The model under review builds one solid part; all positions refer to its coordinate system, in mm. Coordinates: 2 decimals unless noted, no trailing zeros. Order: outer loops, then holes, each group sorted by start corner. A loop starts at its lowest first (then second) coordinate and runs counter-clockwise, first axis right, second up. Notation, with made-up numbers: M -5.75,87.25 L 20.25,87.25 A19 ccw 20.25,93.25 Z; hole C 40,84.5 d7. An arc over 180 degrees is marked long. One line per item, written item: value.
```python
from build123d import *

# Parameters (mm, degrees)
F0_R     = 8.5
F1_DEPTH = 3


with BuildPart() as f1:
    # F0 (on Front) → F1 (new body)
    with BuildSketch(Plane.XZ):
        with BuildLine():
            ThreePointArc((0, 55), (16.109127, 16.109127), (55, 0))
            Line((55, 0), (305, 0))
            ThreePointArc((305, 0), (315.606602, 4.393398), (320, 15))
            Line((320, 15), (320, 100))
            ThreePointArc((320, 100), (315.606602, 110.606602), (305, 115))
            Line((305, 115), (15, 115))
            ThreePointArc((15, 115), (4.393398, 110.606602), (0, 100))
            Line((0, 100), (0, 55))
        make_face()
        with Locations((75, 20)):
            Circle(F0_R, mode=Mode.SUBTRACT)
        with Locations((100, 20)):
            Circle(F0_R, mode=Mode.SUBTRACT)
        with Locations((125, 20)):
            Circle(F0_R, mode=Mode.SUBTRACT)
        with Locations((150, 20)):
            Circle(F0_R, mode=Mode.SUBTRACT)
        with Locations((75, 45)):
            Circle(F0_R, mode=Mode.SUBTRACT)
        with Locations((100, 45)):
            Circle(F0_R, mode=Mode.SUBTRACT)
        with Locations((125, 45)):
            Circle(F0_R, mode=Mode.SUBTRACT)
        with Locations((150, 45)):
            Circle(F0_R, mode=Mode.SUBTRACT)
        with Locations((175, 20)):
            Circle(F0_R, mode=Mode.SUBTRACT)
        with Locations((200, 20)):
            Circle(F0_R, mode=Mode.SUBTRACT)
        with Locations((225, 20)):
            Circle(F0_R, mode=Mode.SUBTRACT)
        with Locations((250, 20)):
            Circle(F0_R, mode=Mode.SUBTRACT)
        with Locations((275, 20)):
            Circle(F0_R, mode=Mode.SUBTRACT)
        with Locations((300, 20)):
            Circle(F0_R, mode=Mode.SUBTRACT)
        with Locations((175, 45)):
            Circle(F0_R, mode=Mode.SUBTRACT)
        with Locations((200, 45)):
            Circle(F0_R, mode=Mode.SUBTRACT)
        with Locations((225, 45)):
            Circle(F0_R, mode=Mode.SUBTRACT)
        with Locations((250, 45)):
            Circle(F0_R, mode=Mode.SUBTRACT)
        with Locations((275, 45)):
            Circle(F0_R, mode=Mode.SUBTRACT)
        with Locations((300, 45)):
            Circle(F0_R, mode=Mode.SUBTRACT)
        with Locations((75, 70)):
            Circle(F0_R, mode=Mode.SUBTRACT)
        with Locations((100, 70)):
            Circle(F0_R, mode=Mode.SUBTRACT)
        with Locations((125, 70)):
            Circle(F0_R, mode=Mode.SUBTRACT)
        with Locations((150, 70)):
            Circle(F0_R, mode=Mode.SUBTRACT)
        with Locations((100, 95)):
            Circle(F0_R, mode=Mode.SUBTRACT)
        with Locations((125, 95)):
            Circle(F0_R, mode=Mode.SUBTRACT)
        with Locations((150, 95)):
            Circle(F0_R, mode=Mode.SUBTRACT)
        with Locations((175, 70)):
            Circle(F0_R, mode=Mode.SUBTRACT)
        with Locations((200, 70)):
            Circle(F0_R, mode=Mode.SUBTRACT)
        with Locations((225, 70)):
            Circle(F0_R, mode=Mode.SUBTRACT)
        with Locations((250, 70)):
            Circle(F0_R, mode=Mode.SUBTRACT)
        with Locations((275, 70)):
            Circle(F0_R, mode=Mode.SUBTRACT)
        with Locations((300, 70)):
            Circle(F0_R, mode=Mode.SUBTRACT)
        with Locations((175, 95)):
            Circle(F0_R, mode=Mode.SUBTRACT)
        with Locations((225, 95)):
            Circle(F0_R, mode=Mode.SUBTRACT)
        with Locations((250, 95)):
            Circle(F0_R, mode=Mode.SUBTRACT)
        with Locations((275, 95)):
            Circle(F0_R, mode=Mode.SUBTRACT)
        with Locations((300, 95)):
            Circle(F0_R, mode=Mode.SUBTRACT)
    extrude(amount=F1_DEPTH)


solid = f1.part
```
(1) For L1, parallel to Z at x = 174.5, y = -2.25; L2, parallel to Z at x = 74.5, y = -1.15; L3, parallel to Z at x = 230, y = -1.1, list the stretches that pass through material, from the lowest coordinate up.
Geometry results:
L1: z = 0 to 11.51, 28.49 to 36.51, 53.49 to 61.51, 78.49 to 86.51, 103.49 to 115
L2: z = 0 to 11.51, 28.49 to 36.51, 53.49 to 61.51, 78.49 to 115
L3: z = 0 to 13.13, 26.87 to 38.13, 51.87 to 63.13, 76.87 to 88.13, 101.87 to 115
(2) We need section C-C, the plane z = 45. Count the separate pieces of the cut face and the enclosed holes in it, plus the area to 3 significant figures.
Geometry results:
separate pieces: 11
enclosed holes: 0
area: 447 mm2
(3) We need section A-A, the plane x = 300. State the section outline as (y, z) points.
Geometry results:
outline: M -3,0 L 0,0 L 0,11.5 L -3,11.5 Z; M -3,28.5 L 0,28.5 L 0,36.5 L -3,36.5 Z; M -3,53.5 L 0,53.5 L 0,61.5 L -3,61.5 Z; M -3,78.5 L 0,78.5 L 0,86.5 L -3,86.5 Z; M -3,103.5 L 0,103.5 L 0,115 L -3,115 Z
(4) Mouldability with a two-part tool opening along X and no side actions: class faces 1 (the cylindrical face through (293.255, -1.479, 39.828)), 2 (the cylindrical face through (15.684, -1.479, 16.539)) as +X half, -X half, draft (parallel to the pull), parting line (faces both ways), or undercut.
Geometry results:
face 1: undercut
face 2: -X half
(5) We need section B-B, the plane x = 200. State the section outline as (y, z) points.
Geometry results:
outline: M -3,0 L 0,0 L 0,11.5 L -3,11.5 Z; M -3,28.5 L 0,28.5 L 0,36.5 L -3,36.5 Z; M -3,53.5 L 0,53.5 L 0,61.5 L -3,61.5 Z; M -3,78.5 L 0,78.5 L 0,115 L -3,115 Z
